Read the model definition and answer for the solid it produces. Units are mm, in the model's axes. Face numbers are marked on the shaded views. A direction names the side the tool comes from. Coordinates: 2 decimals unless noted, no trailing zeros. Order: outer loops, then holes, each group sorted by start corner. A loop starts at its lowest first (then second) coordinate and runs counter-clockwise, first axis right, second up. Notation, with made-up numbers: M 18.5,84.5 L 77.5,84.5 A27 cw 77.5,109.5 Z; hole C -12.75,88 d10. An arc over 180 degrees is marked long. Write each question's results on one line, items separated by ' | '.
```python
from build123d import *

# Parameters (mm, degrees)
SKETCH_W            = 24.4
SKETCH_H            = 10.4
PAD_DEPTH           = 10
PAD_DEPTH_BACK      = 1
SKETCH001_R         = 33.5
POCKET_DEPTH        = 5
POCKET_DEPTH_BACK   = 100
SKETCH002_R         = 2.75
HOLE_DEPTH          = 72.501
HOLE001_D           = 4.5
HOLE001_DEPTH       = 70
HOLE001_CBORE_D     = 8.8
HOLE001_CBORE_DEPTH = 50
HOLE001_TIPS_R      = 2.25
SKETCH006_W         = 27.565709
SKETCH006_H         = 14.558517
PAD001_DEPTH        = 0.5


with BuildPart() as part:
    # Sketch → Pad (new body, two sides)
    with BuildSketch(Plane.XY) as pad_sk:
        with BuildLine():
            Line((-43.4, 21.5), (-23.4, 21.5))
            Line((-23.4, 21.5), (-23.4, 37.5))
            Line((-23.4, 37.5), (36.821733, 37.5))
            ThreePointArc((67.546316, 21.5), (54.142241, 33.260337), (36.821733, 37.5))
            Line((67.546316, 21.5), (86.6, 21.5))
            Line((86.6, 21.5), (86.6, -21.5))
            Line((86.6, -21.5), (67.546316, -21.5))
            ThreePointArc((36.821733, -37.5), (54.142241, -33.260337), (67.546316, -21.5))
            Line((36.821733, -37.5), (-23.4, -37.5))
            Line((-23.4, -37.5), (-23.4, -21.5))
            Line((-23.4, -21.5), (-43.4, -21.5))
            Line((-43.4, -21.5), (-43.4, 21.5))
        make_face()
        with Locations((-12.2, 12.3)):
            Rectangle(SKETCH_W, SKETCH_H, mode=Mode.SUBTRACT)
    extrude(amount=-PAD_DEPTH)
    extrude(pad_sk.sketch, amount=PAD_DEPTH_BACK)

    # Sketch001 → Pocket (cut, two sides)
    with BuildSketch(Plane.XY) as pocket_sk:
        with Locations((36.821733, 0)):
            Circle(SKETCH001_R)
    extrude(amount=-POCKET_DEPTH, mode=Mode.SUBTRACT)
    extrude(pocket_sk.sketch, amount=POCKET_DEPTH_BACK, mode=Mode.SUBTRACT)

    # Sketch002 → Hole (cut, through all)
    with BuildSketch(Plane.XZ.offset(35)):
        with Locations((-38.4, -5)):
            Circle(SKETCH002_R)
        with Locations((81.6, -5)):
            Circle(SKETCH002_R)
    extrude(amount=-HOLE_DEPTH, mode=Mode.SUBTRACT)

    # Hole001
    with Locations(Plane.XZ.offset(37.5)):
        with Locations((-18.25, -5), (-5.75, -5)):
            CounterBoreHole(HOLE001_D / 2, HOLE001_CBORE_D / 2, HOLE001_CBORE_DEPTH, depth=HOLE001_DEPTH)

    # Hole001 tips → Hole001 tip 1 section 0
    with BuildSketch(Plane.XZ.offset(-32.5), mode=Mode.PRIVATE) as hole001_tip_1_s0:
        with Locations((-18.25, -5)):
            Circle(HOLE001_TIPS_R)
    loft([hole001_tip_1_s0.sketch, Vertex(-18.25, 33.851936, -5)], mode=Mode.SUBTRACT)

    # Hole001 tips → Hole001 tip 2 section 0
    with BuildSketch(Plane.XZ.offset(-32.5), mode=Mode.PRIVATE) as hole001_tip_2_s0:
        with Locations((-5.75, -5)):
            Circle(HOLE001_TIPS_R)
    loft([hole001_tip_2_s0.sketch, Vertex(-5.75, 33.851936, -5)], mode=Mode.SUBTRACT)

    # Sketch006 → Pad001 (join)
    with BuildSketch(Plane.XY.offset(0.5)):
        with Locations((-12.99486, 11.748647)):
            Rectangle(SKETCH006_W, SKETCH006_H)
    extrude(amount=PAD001_DEPTH)


solid = part.part
```
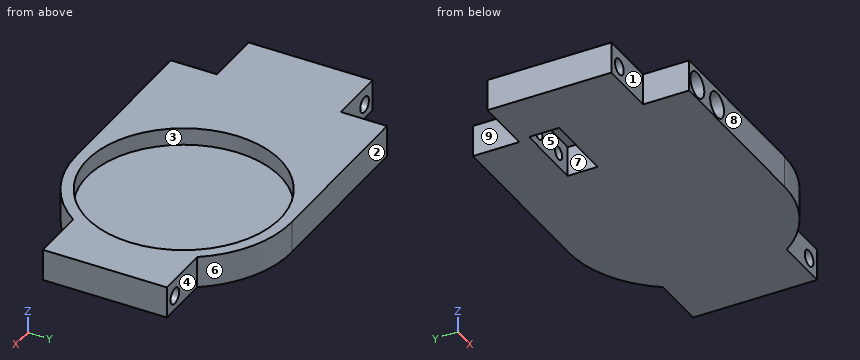
(1) The part is cut by section D-D, the plane x = 59.5. Write down the section's boundary in (y, z).
Conclusion:
outline: M -29.87,-10 L 29.87,-10 L 29.87,1 L 24.66,1 L 24.66,-5 L -24.66,-5 L -24.66,1 L -29.87,1 Z
(2) The mould has two halves that part along X. Classify the marked faces 6, 7, 8 and 9: pulls with the +X half, pulls with the -X half, needs draft (parallel to the pull), parting line crosses it, or undercut.
Conclusion:
face 6: pulls with the +X half | face 7: undercut | face 8: needs draft | face 9: pulls with the -X half
(3) For the marked faces 1, 2, 3, 4 and 5, determine the directions among +Z, -Z, +X, -X, +Y, -Y from which every point of the face is accessible in a straight line to the end or side of a thin tool.
Conclusion:
face 1: +Z, -Z, -X, -Y | face 2: +Z, -Z, +X, -X, +Y | face 3: +Z | face 4: +Z, -Z, +X, +Y | face 5: -Z
(4) The part is cut by section B-B, the plane y = 0. Write down the section's boundary in (x, z), then the cut area to 3 significant figures.
Conclusion:
outline: M -43.4,-10 L 86.6,-10 L 86.6,1 L 70.32,1 L 70.32,-5 L 3.32,-5 L 3.32,1 L -43.4,1 Z; hole C -38.4,-5 d5.5; hole C -18.25,-5 d8.8; hole C -5.75,-5 d8.8; hole C 81.6,-5 d5.5 | area: 859 mm²
(5) Straight lines are drawn through the part: line 1 (Y direction, x = -8, z = 0); line 2 (Z direction, x = -5.75, y = 22); line 3 (X direction, y = -13, z = -4.75). For each, find the intervals that lie inside material, in ascending order.
Conclusion:
line 1: -37.5 to 7.1, 17.5 to 37.5 | line 2: -10 to -7.25, -2.75 to 1 | line 3: -43.4 to -41.14, -35.66 to -22.64, -13.86 to -10.14, -1.36 to 5.95, 67.7 to 78.86, 84.34 to 86.6
(6) The part is cut by section A-A, the plane x = 81.6. Write down the section's boundary in (y, z).
Conclusion:
outline: M -21.5,-10 L 21.5,-10 L 21.5,-7.75 L -21.5,-7.75 Z; M -21.5,-2.25 L 21.5,-2.25 L 21.5,1 L -21.5,1 Z
(7) The part is cut by section C-C, the plane y = 27.5. Write down the section's boundary in (x, z).
Conclusion:
outline: M -23.4,-10 L 62.32,-10 L 62.32,1 L 55.95,1 L 55.95,-5 L 17.69,-5 L 17.69,1 L -23.4,1 Z; hole C -18.25,-5 d4.5; hole C -5.75,-5 d4.5
(8) Given pin 1 (5.5 mm diameter, centred on y = 31.5, z = -4.5, fed in from -X); pin 2 (6 mm diameter, centred on y = -28.5, z = -5.5, fed in from +X); pin 3 (5 mm diameter, centred on x = -15, y = 11.5, fed in from -Z), each flat-ended and moving along its own axis, determine where each tip first touches the part or whether it passes through.
Conclusion:
pin 1: x = -23.4 | pin 2: x = 64.32 | pin 3: z = 0.5
